Input: part model. Units: mm. Frame: model coordinates. Coordinates: 2 decimals unless noted, no trailing zeros. Order: outer loops, then holes, each group sorted by start corner. A loop starts at its lowest first (then second) coordinate and runs counter-clockwise, first axis right, second up. Notation, with made-up numbers: M 10,2 L 37,2 A23 cw 37,13 Z; hole C 14.5,22 d3. An arc over 180 degrees is marked long. Answer in a Markdown table with one row per item.
from build123d import *

# Parameters (mm, degrees)
IZIM5_R   = 0.25
IZIM7_R   = 0.25
RADYUS1_R = 0.4
RADYUS2_R = 0.4


with BuildPart() as part:
    # Çizim3 → Döndür2 (revolve)
    with BuildSketch(Plane(origin=(0, 0, 0), x_dir=(1, 0, 0), z_dir=(0, 1, 0))):
        Polygon((-0.75, -1), (1.75, -1), (1.75, 0), (-1.75, 0), (-1.75, -1), (-1.25, -1), (-1.25, -0.99), (-0.75, -0.99), align=None)
    revolve(axis=Axis((-1.75, 0, 0), (1, 0, 0)))

    # Süpür1: sweep along a path in Çizim4
    with BuildLine(Plane(origin=(0, 0, 0), x_dir=(1, 0, 0), z_dir=(0, 1, 0))) as s_p_r1_path:
        Line((-1.578677494, 0), (-3, 0))
        ThreePointArc((-3, 0), (-3.353553391, -0.146446609), (-3.5, -0.5))
        Line((-3.5, -0.5), (-3.5, -5.5))
    # Çizim5 → Süpür1 (sweep)
    with BuildSketch(Plane.ZY.offset(1.578677494)):
        Circle(IZIM5_R)
    sweep(path=s_p_r1_path.line)

    # Süpür2: sweep along a path in Çizim6
    with BuildLine(Plane(origin=(0, 0, 0), x_dir=(1, 0, 0), z_dir=(0, 1, 0))) as s_p_r2_path:
        Line((1.519396703, 0), (3, 0))
        ThreePointArc((3, 0), (3.353553391, -0.146446609), (3.5, -0.5))
        Line((3.5, -0.5), (3.5, -5.5))
    # Çizim7 → Süpür2 (sweep)
    with BuildSketch(Plane(origin=(1.519396703, 0, 0), x_dir=(0, 0, -1), z_dir=(1, 0, 0))):
        Circle(IZIM7_R)
    sweep(path=s_p_r2_path.line)

    # Radyus1
    # the kernel refuses this fillet: 0.4 mm, written as the material it takes off along each edge
    with BuildSketch(Plane(origin=(1.75, 0, 0), x_dir=(0, 0, 1), z_dir=(0, 1, 0))) as radyus1_piece_1:
        with BuildLine():
            CenterArc((1 - RADYUS1_R, -RADYUS1_R), RADYUS1_R, 0, 90)
            Line((1 - RADYUS1_R, 0), (1 - RADYUS1_R, RADYUS1_R * 0.02))
            Line((1 - RADYUS1_R, RADYUS1_R * 0.02), (1 + RADYUS1_R * 0.02, RADYUS1_R * 0.02))
            Line((1 + RADYUS1_R * 0.02, RADYUS1_R * 0.02), (1 + RADYUS1_R * 0.02, -RADYUS1_R))
            Line((1 + RADYUS1_R * 0.02, -RADYUS1_R), (1, -RADYUS1_R))
        make_face()
    revolve(axis=Axis((1.75, 0, 0), (1, 0, 0)), mode=Mode.SUBTRACT)
    with BuildSketch(Plane(origin=(-0.75, 0, 0), x_dir=(0, 0, 1), z_dir=(0, 1, 0))) as radyus1_piece_2:
        with BuildLine():
            CenterArc((0.6, 0.088881944), RADYUS1_R, 347.161431859, 12.838568141)
            Line((0.99, 0), (0.9978, -0.001777639))
            ThreePointArc((0.9978, -0.001777639), (0.995, -0.008), (1, -0.008))
            Line((1, -0.008), (1.008, 0))
            Line((1.008, 0), (1.008, 0.088881944))
            Line((1.008, 0.088881944), (1, 0.088881944))
        make_face()
    revolve(axis=Axis((-0.75, 0, 0), (1, 0, 0)), mode=Mode.SUBTRACT)

    # Radyus2
    # the kernel refuses this fillet: 0.4 mm, written as the material it takes off along each edge
    with BuildSketch(Plane(origin=(-1.25, 0, 0), x_dir=(0, 0, 1), z_dir=(0, 1, 0))) as radyus2_piece_1:
        with BuildLine():
            CenterArc((0.6, -0.088881944), RADYUS2_R, 0, 12.838568141)
            Line((1, -0.088881944), (1.008, -0.088881944))
            Line((1.008, -0.088881944), (1.008, 0))
            Line((1.008, 0), (1, 0.008))
            ThreePointArc((1, 0.008), (0.995, 0.008), (0.9978, 0.001777639))
            Line((0.9978, 0.001777639), (0.99, 0))
        make_face()
    revolve(axis=Axis((-1.25, 0, 0), (1, 0, 0)), mode=Mode.SUBTRACT)
    with BuildSketch(Plane(origin=(-1.75, 0, 0), x_dir=(0, 0, 1), z_dir=(0, 1, 0))) as radyus2_piece_2:
        with BuildLine():
            CenterArc((1 - RADYUS2_R, RADYUS2_R), RADYUS2_R, 270, 90)
            Line((1 - RADYUS2_R, 0), (1 - RADYUS2_R, -RADYUS2_R * 0.02))
            Line((1 - RADYUS2_R, -RADYUS2_R * 0.02), (1 + RADYUS2_R * 0.02, -RADYUS2_R * 0.02))
            Line((1 + RADYUS2_R * 0.02, -RADYUS2_R * 0.02), (1 + RADYUS2_R * 0.02, RADYUS2_R))
            Line((1 + RADYUS2_R * 0.02, RADYUS2_R), (1, RADYUS2_R))
        make_face()
    revolve(axis=Axis((-1.75, 0, 0), (1, 0, 0)), mode=Mode.SUBTRACT)


solid = part.part
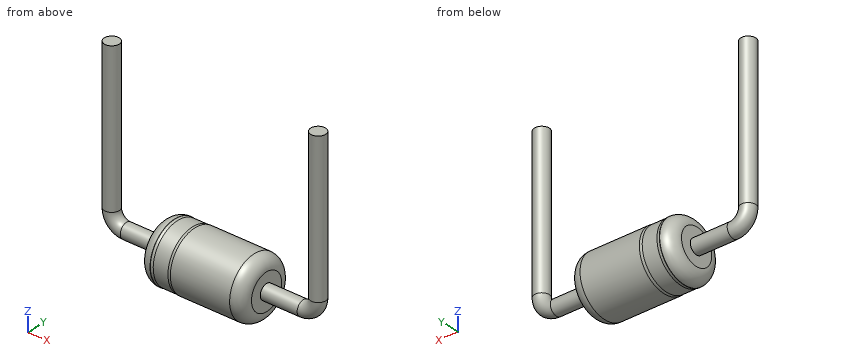
1) Cut plane A-A, the plane z = 2. Output: boundary loops of the cut face in (x, y), and give its area (3 significant figures).
Resolved:
| item | result |
|---|---|
| outline | C -3.5,0 d0.5; C 3.5,0 d0.5 |
| area | 0.393 mm2 |
2) Material intervals for probe 1 along X at (y, z) = (-0.05, 0.75); probe 2 along Z at (x, y) = (0, 0.8); probe 3 along X at (y, z) = (-0.05, 4), sorted ascending.
Resolved:
| item | result |
|---|---|
| probe 1 | x = -3.74 to -3.26, -1.72 to 1.72, 3.26 to 3.74 |
| probe 2 | z = -0.6 to 0.6 |
| probe 3 | x = -3.74 to -3.26, 3.26 to 3.74 |
3) Contact query for flat-ended pins moving along their axis: pin 1 (2 mm diameter, centred on x = -2.5, z = 1.5, fed in from +Y); pin 2 (1 mm diameter, centred on x = -2, y = -0.5, fed in from +Z); pin 3 (3 mm diameter, centred on x = -2.5, z = 1.5, fed in from -Y). Output: stop coordinate, or through.
Resolved:
| item | result |
|---|---|
| pin 1 | stops at y = 0.25 |
| pin 2 | stops at z = 0.9 |
| pin 3 | stops at y = -0.89 |
4) Cut plane C-C, the plane x = 0.75. Output: boundary loops of the cut face in (y, z), and give its area (3 significant figures).
Resolved:
| item | result |
|---|---|
| outline | C 0,0 d2 |
| area | 3.14 mm2 |
5) Cut plane D-D, the plane x = 2. Output: boundary loops of the cut face in (y, z).
Resolved:
| item | result |
|---|---|
| outline | C 0,0 d0.5 |
